For this review, take the finished solid that the model builds, in its own axes (mm). Face numbers are marked on the shaded views. A direction names the side the tool comes from. Coordinates: 2 decimals unless noted, no trailing zeros. Write each loop counter-clockwise with the first axis right and the second up, starting at its lowest first coordinate (ties: lowest second). Pieces come first, ordered by that corner, then holes. Notation, with made-up numbers: M 7,-16 L 21,-16 A15 ccw 21,4 Z; hole C 89,75.25 d1. An arc over 180 degrees is marked long. One line per question, with ' | ' between items.
from build123d import *

# Parameters (mm, degrees)
SKETCH2_W           = 266.7
SKETCH2_H           = 273.05
BOSS_EXTRUDE1_DEPTH = 3.175
SKETCH3_R           = 9.525
CUT_EXTRUDE1_DEPTH  = 4.175
SKETCH4_W           = 76.2
SKETCH4_H           = 76.2
CUT_EXTRUDE2_DEPTH  = 4.175
FILLET2_R           = 6.35
SKETCH5_W           = 177.8
SKETCH5_H           = 3.175
SKETCH5_W_2         = 3.175
SKETCH5_H_2         = 177.8
BOSS_EXTRUDE2_DEPTH = 25.4
CUT_EXTRUDE3_DEPTH  = 267.7
CUT_EXTRUDE4_DEPTH  = 274.05
SKETCH8_R           = 2.54
CUT_EXTRUDE5_DEPTH  = 4.175
SKETCH10_R          = 2.38125
CUT_EXTRUDE6_DEPTH  = 274.05
SKETCH11_R          = 2.413
CUT_EXTRUDE7_DEPTH  = 267.7


with BuildPart() as part:
    # Sketch2 → Boss-Extrude1 (new body)
    with BuildSketch(Plane(origin=(0, 0, 0), x_dir=(1, 0, 0), z_dir=(0, 1, 0))):
        with Locations((133.35, 136.525)):
            Rectangle(SKETCH2_W, SKETCH2_H)
    extrude(amount=BOSS_EXTRUDE1_DEPTH)

    # Sketch3 → Cut-Extrude1 (cut, through all)
    with BuildSketch(Plane(origin=(0, 3.175, 0), x_dir=(1, 0, 0), z_dir=(0, 1, 0))):
        with Locations((133.262465238, 136.525)):
            Circle(SKETCH3_R)
    extrude(amount=-CUT_EXTRUDE1_DEPTH, mode=Mode.SUBTRACT)

    # Sketch4 → Cut-Extrude2 (cut, through all)
    with BuildSketch(Plane(origin=(0, 3.175, 0), x_dir=(1, 0, 0), z_dir=(0, 1, 0))):
        with Locations((64.623665915, 202.110512242)):
            Rectangle(SKETCH4_W, SKETCH4_H)
        with Locations((195.760512242, 202.110512242)):
            Rectangle(SKETCH4_W, SKETCH4_H)
        with Locations((64.623665915, 70.939487758)):
            Rectangle(SKETCH4_W, SKETCH4_H)
        with Locations((195.760512242, 70.939487758)):
            Rectangle(SKETCH4_W, SKETCH4_H)
    extrude(amount=-CUT_EXTRUDE2_DEPTH, mode=Mode.SUBTRACT)

    # Fillet2
    fillet2_edges = [part.edges().sort_by_distance(p)[0] for p in [
        (26.523665915, 1.5875, -164.010512242),
        (26.523665915, 1.5875, -240.210512242),
        (102.723665915, 1.5875, -240.210512242),
        (102.723665915, 1.5875, -164.010512242),
        (157.660512242, 1.5875, -164.010512242),
        (157.660512242, 1.5875, -240.210512242),
        (233.860512242, 1.5875, -240.210512242),
        (233.860512242, 1.5875, -164.010512242),
        (26.523665915, 1.5875, -32.839487758),
        (26.523665915, 1.5875, -109.039487758),
        (102.723665915, 1.5875, -109.039487758),
        (102.723665915, 1.5875, -32.839487758),
        (157.660512242, 1.5875, -32.839487758),
        (157.660512242, 1.5875, -109.039487758),
        (233.860512242, 1.5875, -109.039487758),
        (233.860512242, 1.5875, -32.839487758),
    ]]
    fillet(fillet2_edges, radius=FILLET2_R)

    # Sketch5 → Boss-Extrude2 (add)
    with BuildSketch(Plane(origin=(0, 3.175, 0), x_dir=(1, 0, 0), z_dir=(0, 1, 0))):
        with Locations((133.35, 271.4625)):
            Rectangle(SKETCH5_W, SKETCH5_H)
        with Locations((133.35, 1.5875)):
            Rectangle(SKETCH5_W, SKETCH5_H)
        with Locations((265.1125, 136.525)):
            Rectangle(SKETCH5_W_2, SKETCH5_H_2)
        with Locations((1.5875, 136.525)):
            Rectangle(SKETCH5_W_2, SKETCH5_H_2)
    extrude(amount=BOSS_EXTRUDE2_DEPTH)

    # Sketch6 → Cut-Extrude3 (cut, through all)
    with BuildSketch(Plane(origin=(266.7, 0, 0), x_dir=(0, 0, -1), z_dir=(1, 0, 0))):
        Polygon((47.625, 3.175), (73.025, 28.575), (47.625, 28.575), align=None)
        Polygon((225.425, 3.175), (200.025, 28.575), (225.425, 28.575), align=None)
    extrude(amount=-CUT_EXTRUDE3_DEPTH, mode=Mode.SUBTRACT)

    # Sketch7 → Cut-Extrude4 (cut, through all)
    with BuildSketch(Plane.XY):
        Polygon((44.45, 3.175), (69.85, 28.575), (44.45, 28.575), align=None)
        Polygon((222.25, 3.175), (196.85, 28.575), (222.25, 28.575), align=None)
    extrude(amount=-CUT_EXTRUDE4_DEPTH, mode=Mode.SUBTRACT)

    # Sketch8 → Cut-Extrude5 (cut, through all)
    with BuildSketch(Plane(origin=(0, 3.175, 0), x_dir=(1, 0, 0), z_dir=(0, 1, 0))):
        with Locations((151.118665238, 136.525)):
            Circle(SKETCH8_R)
        with Locations((115.406265238, 135.851510726)):
            Circle(SKETCH8_R)
    extrude(amount=-CUT_EXTRUDE5_DEPTH, mode=Mode.SUBTRACT)

    # Sketch10 → Cut-Extrude6 (cut, through all)
    with BuildSketch(Plane.XY):
        with Locations((133.35, 15.875)):
            Circle(SKETCH10_R)
        with Locations((158.75, 15.875)):
            Circle(SKETCH10_R)
        with Locations((107.95, 15.875)):
            Circle(SKETCH10_R)
        with Locations((82.55, 15.875)):
            Circle(SKETCH10_R)
        with Locations((184.15, 15.875)):
            Circle(SKETCH10_R)
    extrude(amount=-CUT_EXTRUDE6_DEPTH, mode=Mode.SUBTRACT)

    # Sketch11 → Cut-Extrude7 (cut, through all)
    with BuildSketch(Plane(origin=(266.7, 0, 0), x_dir=(0, 0, -1), z_dir=(1, 0, 0))):
        with Locations((136.4488, 15.875)):
            Circle(SKETCH11_R)
        with Locations((111.0488, 15.875)):
            Circle(SKETCH11_R)
        with Locations((85.6488, 15.875)):
            Circle(SKETCH11_R)
        with Locations((161.8488, 15.875)):
            Circle(SKETCH11_R)
        with Locations((187.2488, 15.875)):
            Circle(SKETCH11_R)
    extrude(amount=-CUT_EXTRUDE7_DEPTH, mode=Mode.SUBTRACT)


solid = part.part
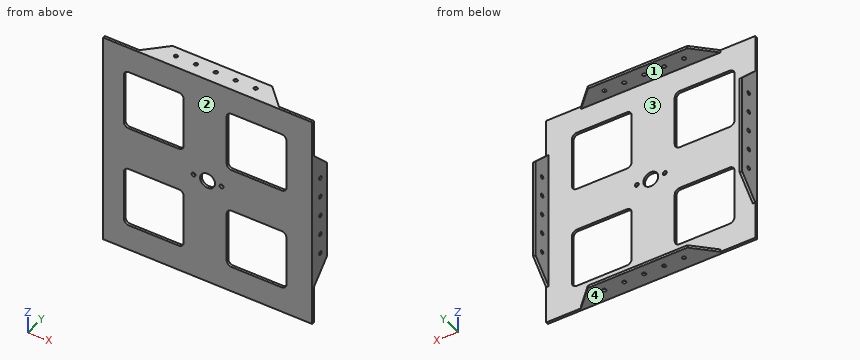
1. Draft analysis for pull direction X (two halves, no side actions). For the marked faces 3 and 4, state which applies: pulls with the +X half, pulls with the -X half, needs draft (parallel to the pull), parting line crosses it, or undercut.
Computed values:
face 3: undercut | face 4: needs draft
2. Take a section at C-C on y = 8.25. State the section outline as (x, z) points (3 decimals), plus the area to 3 significant figures.
Computed values:
outline: M 0,-220.35 L 3.175,-220.35 L 3.175,-52.7 L 0,-52.7 Z; M 49.525,-273.05 L 217.175,-273.05 L 217.175,-269.875 L 49.525,-269.875 Z; M 49.525,-3.175 L 217.175,-3.175 L 217.175,0 L 49.525,0 Z; M 263.525,-220.35 L 266.7,-220.35 L 266.7,-52.7 L 263.525,-52.7 Z | area: 2,130 mm2
3. Take a section at D-D on z = -28. State the section outline as (x, y) points (3 decimals), plus the area to 3 significant figures.
Computed values:
outline: M 0,0 L 266.7,0 L 266.7,3.175 L 0,3.175 Z | area: 847 mm2
4. Take a section at A-A on z = -80. State the section outline as (x, y) points (3 decimals).
Computed values:
outline: M 0,0 L 26.524,0 L 26.524,3.175 L 3.175,3.175 L 3.175,28.575 L 0,28.575 Z; M 102.724,0 L 157.661,0 L 157.661,3.175 L 102.724,3.175 Z; M 233.861,0 L 266.7,0 L 266.7,28.575 L 263.525,28.575 L 263.525,3.175 L 233.861,3.175 Z
5. Machinability: for the marked faces 1 and 2, which of the approach directions +Z, -Z, +X, -X, +Y, -Y give a long, thin tool a straight path to every point of the face, cutting with its end or side? Answer none if there is none.
Computed values:
face 1: +X, -X, +Y | face 2: +Z, -Z, +X, -X, -Y
6. Take a section at B-B on x = 202. State the section outline as (y, z) points (3 decimals).
Computed values:
outline: M 0,-273.05 L 23.425,-273.05 L 23.425,-269.875 L 3.175,-269.875 L 3.175,-240.211 L 0,-240.211 Z; M 0,-164.011 L 3.175,-164.011 L 3.175,-109.039 L 0,-109.039 Z; M 0,-32.839 L 3.175,-32.839 L 3.175,-3.175 L 23.425,-3.175 L 23.425,0 L 0,0 Z
7. For line 1 along X through (y, z) = (1.5, -52.5); line 2 along Z through (x, y) = (100, 20.75) (3 decimals); line 3 along X through (y, z) = (20.25, -67.5) (3 decimals), list the stretches that pass through material, from the lowest coordinate up.
Computed values:
line 1: x = 0 to 26.52, 102.72 to 157.66, 233.86 to 266.7 | line 2: z = -273.05 to -269.875, -3.175 to 0 | line 3: x = 0 to 3.175, 263.525 to 266.7
